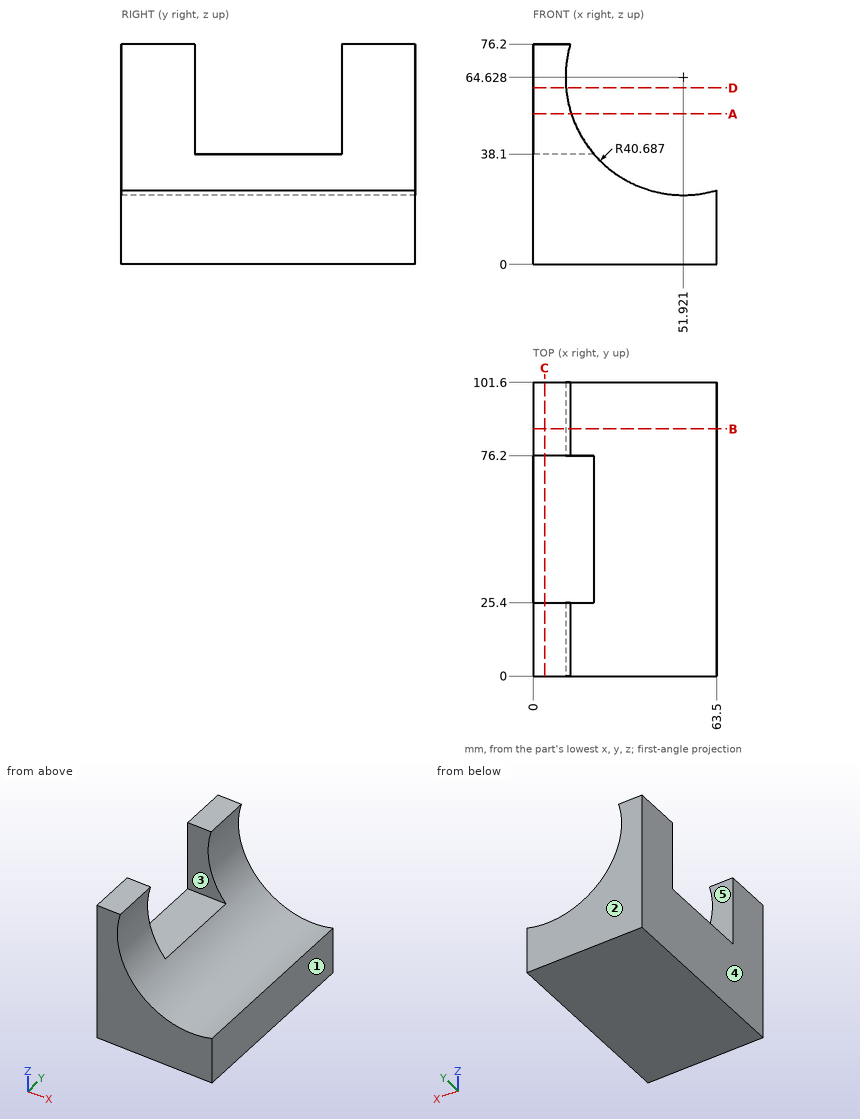
The drawing under review shows one solid part. Ordinate dimensions are in mm from its lowest x, y, z. A direction names the side the tool comes from. Round coordinates to 2 decimals unless told otherwise and drop trailing zeros. Loops run counter-clockwise (first coordinate to the right, second up) from the corner with the lowest first, then second, coordinate; pieces in that order, holes last.
Item 1: Take a section at C-C (x = 4). Write out the cut boundary in (y, z).
Determined:
outline: (0, 0) - (101.6, 0) - (101.6, 76.2) - (76.2, 76.2) - (76.2, 38.1) - (25.4, 38.1) - (25.4, 76.2) - (0, 76.2) - close
Item 2: Clearance check with flat-ended pins moving along their axes: pin 1 Ø10.5 at (x, y) = (9, 48) entering from +Z; pin 2 Ø23 at (x, z) = (5.5, 59) entering from -Y. State where each tip first meets the part, or that it passes through.
Determined:
pin 1: stops at z = 38.1
pin 2: stops at y = 0
Item 3: Take a section at A-A (z = 52). Write out the cut boundary in (x, y).
Determined:
outline: (0, 0) - (13.24, 0) - (13.24, 25.4) - (0, 25.4) - close; (0, 76.2) - (13.24, 76.2) - (13.24, 101.6) - (0, 101.6) - close
Item 4: Mouldability with a two-part tool opening along Y and no side actions: class the marked faces 1, 2 and 3 as released by +Y, released by -Y, zero draft, split by the parting line, or undercut.
Determined:
face 1: zero draft
face 2: released by +Y
face 3: undercut
Item 5: Take a section at B-B (y = 85.5). Write out the cut boundary in (x, z) (1 decimal), then the cut area to 3 significant figures.
Determined:
outline: (0, 0) - (63.5, 0) - (63.5, 25.6) arc R40.7 cw to (12.9, 76.2) - (0, 76.2) - close
area: 2,480 mm2
Item 6: Take a section at D-D (z = 61). Write out the cut boundary in (x, y), then the cut area to 3 significant figures.
Determined:
outline: (0, 0) - (11.4, 0) - (11.4, 25.4) - (0, 25.4) - close; (0, 76.2) - (11.4, 76.2) - (11.4, 101.6) - (0, 101.6) - close
area: 579 mm2
Item 7: For line 1 (Y direction, x = 11.5, z = 42); line 2 (X direction, y = 15, z = 64); line 3 (X direction, y = 11, z = 61), list the stretches that pass through material, from the lowest coordinate up.
Determined:
line 1: y = 0 to 25.4, 76.2 to 101.6
line 2: x = 0 to 11.24
line 3: x = 0 to 11.4
Item 8: For the marked faces 4 and 5, list the 3-axis set-ups (+Z, -Z, +X, -X, +Y, -Y) from which the entire face can be reached by the end or side of a thin tool; tool diameter is ignored.
Determined:
face 4: +Z, -Z, -X, +Y, -Y
face 5: +Z, +X, -X
